Can you work these out from the model? Positions are in its coordinate system, mm. Give positions to 0.01 mm unless a question says otherwise; leave off trailing zeros. Order: outer loops, then holes, each group sorted by start corner. A loop starts at its lowest first (then second) coordinate and runs counter-clockwise, first axis right, second up. Notation, with made-up numbers: M -21,2.25 L 14,2.25 A18 cw 14,12.25 Z; hole C 69,25.25 d7. An arc over 180 degrees is marked long. One line per question, with ' | ' between items. Start each with the question number.
1) If we section it at C-C, the plane x = 3.75: State how many separate pieces and enclosed holes the cut face has, plus the area to 3 significant figures.
2) If we section it at B-B, the plane z = -12: Please give me the cut outline in (x, y), plus the area to 3 significant figures.
3) Please list where these lines run through material, in increasing order: line 1 along Y through (x, z) = (2, -73); line 2 along Y through (x, z) = (5.75, -71.5); line 3 along Z through (x, y) = (6, 44). Write a range as [from, to].
4) If we section it at A-A, the plane y = 0: Please give me the cut outline in (x, z).
5) If we section it at D-D, the plane y = 75.05: Please give me the cut outline in (x, z).
6) I'm going to push flat-ended pins straight in: pin 1 Ø1 at (x, z) = (4.5, 53) entering from -Y; pin 2 Ø1.9 at (x, y) = (2, 60) entering from -Z; pin 3 Ø1.5 at (x, y) = (5, 56.5) entering from +Z. Where does each tip first touch, or does it pass through?
```python
from build123d import *

# Parameters (mm, degrees)
SKETCH1_R           = 36.5125
BOSS_EXTRUDE1_DEPTH = 6.35
SKETCH3_R           = 2.5
CUT_EXTRUDE1_DEPTH  = 114.315146825
CIRPATTERN1_COUNT   = 8
SKETCH4_R           = 2.5
CUT_EXTRUDE4_DEPTH  = 114.315146825


with BuildPart() as part:
    # Sketch1 → Boss-Extrude1 (new body)
    with BuildSketch(Plane(origin=(0, 0, 0), x_dir=(0, 0, -1), z_dir=(1, 0, 0))):
        with BuildLine():
            Line((77.95, 80), (0, 80))
            ThreePointArc((0, 80), (-37.416573868, -70.710678119), (66.143782777, 45))
            Line((66.143782777, 45), (77.95, 45))
            Line((77.95, 45), (77.95, 80))
        make_face()
        Circle(SKETCH1_R, mode=Mode.SUBTRACT)
    extrude(amount=BOSS_EXTRUDE1_DEPTH)

    # Sketch3 → Cut-Extrude1 (cut, through all)
    with BuildSketch(Plane(origin=(6.35, 0, 0), x_dir=(0, 0, -1), z_dir=(1, 0, 0))):
        with Locations((11.979044202, 75.05)):
            Circle(SKETCH3_R)
    cut_extrude1 = extrude(amount=-CUT_EXTRUDE1_DEPTH, mode=Mode.SUBTRACT)

    # CirPattern1: Cut-Extrude1 ×8 about axis, 1 skipped
    cirpattern1_axis = Axis((0, 0, 0), (1, 0, 0))
    add([cut_extrude1.rotate(cirpattern1_axis, i * 360 / CIRPATTERN1_COUNT) for i in range(1, CIRPATTERN1_COUNT) if i not in (7,)], mode=Mode.SUBTRACT)

    # Sketch4 → Cut-Extrude4 (cut, through all)
    with BuildSketch(Plane(origin=(6.35, 0, 0), x_dir=(0, 0, -1), z_dir=(1, 0, 0))):
        with Locations((36, 75.05)):
            Circle(SKETCH4_R)
        with Locations((73, 75.05)):
            Circle(SKETCH4_R)
        with Locations((73, 49.95)):
            Circle(SKETCH4_R)
        with Locations((61.665635624, 44.422397314)):
            Circle(SKETCH4_R)
    extrude(amount=-CUT_EXTRUDE4_DEPTH, mode=Mode.SUBTRACT)


solid = part.part
```
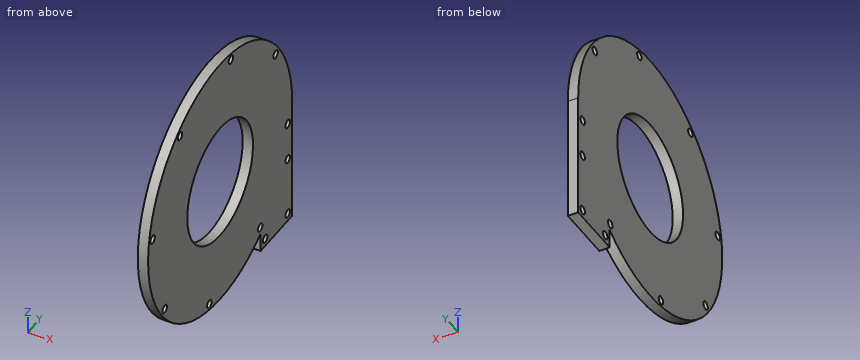
Results found:
1) separate pieces: 1 | enclosed holes: 12 | area: 16,800 mm²
2) outline: M 0,-79.09 L 6.35,-79.09 L 6.35,-34.48 L 0,-34.48 Z; M 0,34.48 L 6.35,34.48 L 6.35,72.55 L 0,72.55 Z; M 0,77.55 L 6.35,77.55 L 6.35,80 L 0,80 Z | area: 541 mm²
3) line 1: y = [-32.73, -13.41], [-10.55, 32.73], [45, 47.45], [52.45, 72.55], [77.55, 80] | line 2: y = [-35.89, 35.89], [45, 47.95], [51.95, 73.05], [77.05, 80] | line 3: z = [-66.81, -64.13], [-59.2, 66.81]
4) outline: M 0,-80 L 6.35,-80 L 6.35,-36.51 L 0,-36.51 Z; M 0,36.51 L 6.35,36.51 L 6.35,80 L 0,80 Z
5) outline: M 0,-77.95 L 6.35,-77.95 L 6.35,-75.5 L 0,-75.5 Z; M 0,-70.5 L 6.35,-70.5 L 6.35,-38.5 L 0,-38.5 Z; M 0,-33.5 L 6.35,-33.5 L 6.35,-14.48 L 0,-14.48 Z; M 0,-9.48 L 6.35,-9.48 L 6.35,27.7 L 0,27.7 Z
6) pin 1: stops at y = -60.36 | pin 2: stops at z = -77.95 | pin 3: stops at z = 57.38
